Autodesk Inventor part; units mm, degrees
ref_plane "YZ Plane" through (0, 0, 0) normal (1, 0, 0) x (0, 1, 0)
ref_plane "XZ Plane" through (0, 0, 0) normal (0, 1, 0) x (-1, 0, 0)
ref_plane "XY Plane" through (0, 0, 0) normal (0, 0, 1) x (1, 0, 0)
sketch "Sketch2" plane through (0, 0, 0) normal (0, 1, 0) x (-1, 0, 0)
  line L0 (15, 20.15) -> (20.15, 15)
  line L1 (20.15, 15) -> (20.15, -15)
  line L2 (20.15, -15) -> (15, -20.15)
  line L3 (15, -20.15) -> (-15, -20.15)
  line L4 (-15, -20.15) -> (-20.15, -15)
  line L5 (-20.15, -15) -> (-20.15, 15)
  line L6 (-20.15, 15) -> (-15, 20.15)
  line L7 (-15, 20.15) -> (15, 20.15)
  point P0 (0, 0)
  point P1 (20.15, 0)
  point P2 (0, -20.15)
  dimension "d2" = 30
  dimension "d3" = 40.3
  dimension "d4" = 135
extrude "Extrusion1" add sketch "Sketch2" along normal mid plane 34
sketch "Sketch7" plane through (0, 17, 0) normal (0, 1, 0) x (1, 0, 0)
  circle A0 centre (0, 0) radius 11
  dimension "d27" = 22
extrude "Extrusion3" add sketch "Sketch7" along normal blind 2
sketch "Sketch8" plane through (0, 19, 0) normal (0, 1, 0) x (1, 0, 0)
  circle A0 centre (0, 0) radius 4
  dimension "d30" = 8
extrude "Extrusion4" cut sketch "Sketch8" against normal blind 1
sketch "Sketch9" plane through (0, 18, 0) normal (0, 1, 0) x (1, 0, 0)
  circle A0 centre (0, 0) radius 3.175
  dimension "d33" = 6.35
extrude "Extrusion5" add sketch "Sketch9" along normal blind 23
sketch "Sketch10" plane through (-15, 17, 20.15) normal (0, 0, 1) x (1, 0, 0)
  line L0 (30, 0) -> (30, -34)
  line L1 (0, 0) -> (30, 0)
  line L2 (0, -34) -> (0, 0)
  line L3 (30, -34) -> (0, -34)
  line L4 (0, 0) -> (30, 0)
  line L5 (30, 0) -> (30, -10)
  line L6 (30, -10) -> (0, -10)
  line L7 (0, -10) -> (0, 0)
  line L8 (0, 0) -> (30, -10) construction
  line L9 (30, 0) -> (0, -10) construction
  line L10 (0, -24) -> (30, -24)
  line L11 (30, -24) -> (30, -34)
  line L12 (30, -34) -> (0, -34)
  line L13 (0, -34) -> (0, -24)
  line L14 (0, -24) -> (30, -34) construction
  line L15 (30, -24) -> (0, -34) construction
  line L16 (0, 0) -> (30, 0)
  point P0 (15, -17)
  point P1 (15, -5)
  point P2 (15, -29)
  dimension "d36" = 10
  dimension "d37" = 10
extrude "Extrusion6" add sketch "Sketch10" along normal blind 1 contours L0 L6 L2 L1 | L0 L3 L2 L10
mirror "Mirror1" about plane through (0, 0, 0) normal (0, 0, 1) of "Extrusion6"
sketch "Sketch11" plane through (20.15, -17, -15) normal (1, 0, 0) x (0, 0, -1)
  line L0 (0, 34) -> (0, 0)
  line L1 (-30, 34) -> (0, 34)
  line L2 (-30, 34) -> (-30, 0)
  line L3 (0, 0) -> (-30, 0)
  line L4 (-30, 34) -> (0, 34)
  line L5 (0, 34) -> (0, 24)
  line L6 (0, 24) -> (-30, 24)
  line L7 (-30, 24) -> (-30, 34)
  line L8 (-30, 34) -> (0, 24) construction
  line L9 (0, 34) -> (-30, 24) construction
  line L10 (-30, 10) -> (0, 10)
  line L11 (0, 10) -> (0, 0)
  line L12 (0, 0) -> (-30, 0)
  line L13 (-30, 0) -> (-30, 10)
  line L14 (-30, 10) -> (0, 0) construction
  line L15 (0, 10) -> (-30, 0) construction
  line L16 (-30, 34) -> (0, 34)
  point P0 (-15, 17)
  point P1 (-15, 29)
  point P2 (-15, 5)
  dimension "d40" = 10
extrude "Extrusion7" add sketch "Sketch11" along normal blind 1 contours L0 L6 L2 L1 | L0 L3 L2 L10
mirror "Mirror2" about plane through (0, 0, 0) normal (1, 0, 0) of "Extrusion7"
sketch "Sketch12" plane through (-15, -7, 20.15) normal (-0.7071, 0, 0.7071) x (0.7071, 0, 0.7071)
  line L0 (0, -10) -> (0, 0)
  line L1 (0, 0) -> (0, 14)
  line L2 (0, 14) -> (0, 24)
  line L3 (-7.2832, 24) -> (0, 24)
  line L4 (-7.2832, 24) -> (-7.2832, 14)
  line L5 (-7.2832, 14) -> (-7.2832, 0)
  line L6 (-7.2832, 0) -> (-7.2832, -10)
  line L7 (0, -10) -> (-7.2832, -10)
  line L8 (-7.2832, 24) -> (0, 24)
  line L9 (0, 24) -> (0, 14)
  line L10 (0, 14) -> (-7.2832, 14)
  line L11 (-7.2832, 14) -> (-7.2832, 24)
  line L12 (-7.2832, 24) -> (0, 14) construction
  line L13 (0, 24) -> (-7.2832, 14) construction
  line L14 (-7.2832, 0) -> (0, 0)
  line L15 (0, 0) -> (0, -10)
  line L16 (0, -10) -> (-7.2832, -10)
  line L17 (-7.2832, -10) -> (-7.2832, 0)
  line L18 (-7.2832, 0) -> (0, -10) construction
  line L19 (0, 0) -> (-7.2832, -10) construction
  line L20 (-7.2832, 24) -> (0, 24)
  line L21 (0, -10) -> (-7.2832, -10)
  point P0 (-3.6416, 7)
  point P1 (-3.6416, 19)
  point P2 (-3.6416, -5)
  dimension "d43" = 10
  dimension "d44" = 10
extrude "Extrusion8" add sketch "Sketch12" along normal blind 1 contours L7 L6 L14 L0 | L10 L4 L3 L2
sketch "Sketch14" plane through (-15, 7, 21.15) normal (-1, 0, 0) x (0, 0, 1)
  line L0 (-1, 0) -> (-1, 10)
  line L1 (-1, 0) -> (0, 0)
  line L2 (0, 10) -> (0, 0)
  line L3 (-1, 10) -> (0, 10)
  line L4 (-1, -24) -> (-1, -14)
  line L5 (-1, -24) -> (0, -24)
  line L6 (0, -14) -> (0, -24)
  line L7 (-1, -14) -> (0, -14)
  point P0 (-21.15, -7)
extrude "Extrusion9" add sketch "Sketch14" along normal up to surface surface through (-18.2821, 12, 18.2821) normal (-0.7071, 0, 0.7071)
sketch "Sketch15" plane through (-21.15, 7, 15) normal (0, 0, 1) x (1, 0, 0)
  line L0 (1, 10) -> (1, 0)
  line L1 (1, 10) -> (0, 10)
  line L2 (0, 10) -> (0, 0)
  line L3 (1, 0) -> (0, 0)
  line L4 (1, -14) -> (1, -24)
  line L5 (1, -14) -> (0, -14)
  line L6 (0, -14) -> (0, -24)
  line L7 (1, -24) -> (0, -24)
  point P0 (21.15, -7)
extrude "Extrusion10" add sketch "Sketch15" along normal up to surface surface through (-18.2821, -12, 18.2821) normal (-0.7071, 0, 0.7071)
mirror "Mirror3" about plane through (0, 0, 0) normal (1, 0, 0) of "Extrusion8", "Extrusion9", "Extrusion10"
mirror "Mirror4" about plane through (0, 0, 0) normal (0, 0, 1) of "Extrusion8", "Extrusion9", "Extrusion10", "Mirror3"
sketch "Sketch17" plane through (0, 17, 0) normal (0, 1, 0) x (1, 0, 0)
  line L0 (-21.15, -15.4142) -> (-15.4142, -21.15)
  line L1 (-15.4142, -21.15) -> (15.4142, -21.15)
  line L2 (21.15, -15.4142) -> (15.4142, -21.15)
  line L3 (21.15, -15.4142) -> (21.15, 15.4142)
  line L4 (21.15, 15.4142) -> (15.4142, 21.15)
  line L5 (15.4142, 21.15) -> (-15.4142, 21.15)
  line L6 (-21.15, 15.4142) -> (-15.4142, 21.15)
  line L7 (-21.15, 15.4142) -> (-21.15, -15.4142)
  circle A0 centre (0, 0) radius 11
  circle A1 centre (-15.5, -15.5) radius 1.5
  circle A2 centre (-15.5, 15.5) radius 1.5
  circle A3 centre (15.5, 15.5) radius 1.5
  circle A4 centre (15.5, -15.5) radius 1.5
  dimension "d53" = 3
  dimension "d54" = 31
  dimension "d55" = 31
  dimension "d57" = 15.5
  dimension "d66" = 15.5
hole "Hole3" at (-15.5, 17, 15.5) at (-15.5, 17, -15.5) at (15.5, 17, -15.5) at (15.5, 17, 15.5) direction (0, -1, 0) diameter 3 depth 4.5
sketch "Sketch19" plane through (0, 41, 0) normal (0, 1, 0) x (1, 0, 0)
  circle A0 centre (0, 0) radius 3.175
  circle A1 centre (0, 0) radius 3.175
  line L0 (-2.8853, -1.325) -> (2.8853, -1.325)
  dimension "d69" = 4.5
extrude "Extrusion12" cut sketch "Sketch19" against normal blind 15 contours L0 A0 picked at (0, -1.9417)
ref_plane "Work Plane1" through (0, 0, 0) normal (1, 0, 0) x (0, 1, 0)
ref_plane "Work Plane2" through (0, 0, 0) normal (-1, 0, 0) x (0, 1, 0)
ref_plane "Work Plane3" through (0, 0, 0) normal (-1, 0, 0) x (0, 1, 0)
properties part number "Motor_paso"
Design review of the part built by this model. Coordinates are the model's own, in mm. A direction names the side the tool comes from. Give positions to 0.01 mm unless a question says otherwise; leave off trailing zeros. Loops run counter-clockwise (first coordinate to the right, second up) from the corner with the lowest first, then second, coordinate; pieces in that order, holes last. Notation, with made-up numbers: (-24, 9.5) - (28, 9.5) arc R18 cw to (28, 14.5) - close; hole circle Ø10 at (46, -39.5). An arc over 180 degrees is marked (long way). Write item = value, one per line.
1) Draft analysis for pull direction Y (two halves, no side actions). For faces 6 (the face through (-1.4, -7, -20.5)), 7 (the face through (-0.69, 29.34, -3.1)), 8 (the face through (15, 12.5, 15)), state which applies: +Y half, -Y half, draft (parallel to the pull), parting line (faces both ways), or undercut.
Result sheet:
face_6 = undercut
face_7 = draft
face_8 = +Y half
2) Tool access review of faces 1 (the face through (-18.242, 12.07, -18.322)), 2 (the face through (0, 0, -20.15)), 3 (the face through (15, 12.5, -16)), 4 (the face through (17.61, -0.1, 17.54)), 5 (the face through (-21.15, -12, 0)): name each direction out of +Z, -Z, +X, -X, +Y, -Y from which nothing blocks a thin tool from reaching the whole face with its end or side.
Result sheet:
face_1 = -Z, -X, +Y, -Y
face_2 = -Z, +X, -X
face_3 = +Y
face_4 = +Z, +X
face_5 = +Z, -Z, -X, +Y, -Y
3) To check wall thickness, follow line 1 (Z direction, x = 0, y = 18.65) (3 decimals); line 2 (X direction, y = 15.1, z = -15.5); line 3 (Z direction, x = -15, y = 14). State the ranges of each line that lie inside material, in increasing order.
Result sheet:
line_1 = -11 to -4, -3.175 to 3.175, 4 to 11
line_2 = -21.06 to -17, -14 to 14, 17 to 21.06
line_3 = -21.15 to -16.91, -14.09 to 14.09, 16.91 to 21.15
4) Take a section at C-C on y = 10. State the section outline as (x, z) points, and give its area (3 significant figures).
Result sheet:
outline = (-21.15, -15.41) - (-15.41, -21.15) - (15.41, -21.15) - (21.15, -15.41) - (21.15, 15.41) - (15.41, 21.15) - (-15.41, 21.15) - (-21.15, 15.41) - close
area = 1,720 mm2
5) Clearance check with flat-ended pins moving along their axes: pin 1 Ø2 at (x, z) = (0, 2.5) entering from +Y; pin 2 Ø11 at (x, y) = (-5.5, 0) entering from -Z; pin 3 Ø5 at (x, z) = (-15.5, -15.5) entering from +Y. State where each tip first meets the part, or that it passes through.
Result sheet:
pin_1 = 26
pin_2 = -20.15
pin_3 = 17
6) Take a section at B-B on x = 0. State the section outline as (y, z) points (3 decimals).
Result sheet:
outline = (-17, -21.15) - (-7, -21.15) - (-7, -20.15) - (7, -20.15) - (7, -21.15) - (17, -21.15) - (17, -11) - (19, -11) - (19, -4) - (18, -4) - (18, -3.175) - (41, -3.175) - (41, 1.325) - (26, 1.325) - (26, 3.175) - (18, 3.175) - (18, 4) - (19, 4) - (19, 11) - (17, 11) - (17, 21.15) - (7, 21.15) - (7, 20.15) - (-7, 20.15) - (-7, 21.15) - (-17, 21.15) - close
7) Take a section at A-A on z = 12. State the section outline as (x, y) points, and give its area (3 significant figures).
Result sheet:
outline = (-21.15, -17) - (21.15, -17) - (21.15, -7) - (20.15, -7) - (20.15, 7) - (21.15, 7) - (21.15, 17) - (-21.15, 17) - (-21.15, 7) - (-20.15, 7) - (-20.15, -7) - (-21.15, -7) - close
area = 1,410 mm2
8) Take a section at D-D on z = 0. State the section outline as (x, y) points (3 decimals), and give its area (3 significant figures).
Result sheet:
outline = (-21.15, -17) - (21.15, -17) - (21.15, -7) - (20.15, -7) - (20.15, 7) - (21.15, 7) - (21.15, 17) - (11, 17) - (11, 19) - (4, 19) - (4, 18) - (3.175, 18) - (3.175, 41) - (-3.175, 41) - (-3.175, 18) - (-4, 18) - (-4, 19) - (-11, 19) - (-11, 17) - (-21.15, 17) - (-21.15, 7) - (-20.15, 7) - (-20.15, -7) - (-21.15, -7) - close
area = 1,590 mm2
